Input: part model. Units: mm. Frame: model coordinates. Coordinates: 2 decimals unless noted, no trailing zeros. Loops run counter-clockwise (first coordinate to the right, second up) from the corner with the lowest first, then second, coordinate; pieces in that order, holes last.
```python
from build123d import *

# Parameters (mm, degrees)
SKETCH093_W      = 26
SKETCH093_H      = 70
EXTRUDE081_DEPTH = 1
SKETCH_W         = 45
SKETCH_H         = 66
EXTRUDE_DEPTH    = 2


with BuildPart() as extrude081:
    # Sketch093 → Extrude081 (new body, symmetric)
    with BuildSketch(Plane.XY.offset(-22)):
        with Locations((62, 50)):
            Rectangle(SKETCH093_W, SKETCH093_H)
    extrude(amount=EXTRUDE081_DEPTH, both=True)


with BuildPart() as cut012:
    # Sketch → Extrude (new body)
    with BuildSketch(Plane(origin=(0, 0, -22), x_dir=(1, 0, 0), z_dir=(0, 0, -1))):
        Polygon((-7, 2), (81, 2), (81, -102), (-7, -102), (-7, -100), (-2, -100), (-2, -93.5), (-3, -93.5), (-3, -9), (-2, -9), (-2, 0), (-7, 0), align=None)
        with Locations((20.5, -52)):
            Rectangle(SKETCH_W, SKETCH_H, mode=Mode.SUBTRACT)
    extrude(amount=EXTRUDE_DEPTH)

    # Cut012: cut Extrude081
    add(extrude081.part, mode=Mode.SUBTRACT)


solid = cut012.part
```
Item 1: Line query: L1, parallel to X at y = 20.5, z = -22.05; L2, parallel to Y at x = 6, z = -23.2; L3, parallel to X at y = 26, z = -23.85. Output: solid intervals per line, ascending.
Result:
L1: x = -3 to -2, 43 to 49, 75 to 81
L2: y = -2 to 19, 85 to 102
L3: x = -3 to -2, 43 to 81
Item 2: Section query B-B (z = -23.55). Output: boundary loops of the cut face in (x, y).
Result:
outline: (-7, -2) - (81, -2) - (81, 102) - (-7, 102) - (-7, 100) - (-2, 100) - (-2, 93.5) - (-3, 93.5) - (-3, 9) - (-2, 9) - (-2, 0) - (-7, 0) - close; hole (-2, 19) - (43, 19) - (43, 85) - (-2, 85) - close
Item 3: Mould query, pull axis Y, two halves, no side actions, for faces 1 (the face through (62, 50, -23)), 2 (the face through (47, 38, -22)). Classes: +Y half, -Y half, draft (parallel to the pull), parting line (faces both ways), or undercut.
Result:
face 1: undercut
face 2: draft
Item 4: Contact query for flat-ended pins moving along their axis: P1, Ø6, axis at x = 64, y = 44.5, coming from the +Z side; P2, Ø0.5, axis at y = 66.5, z = -22.5, coming from the -X side; P3, Ø0.6, axis at y = 95.5, z = -22.5, coming from the -X side. Output: stop coordinate, or through.
Result:
P1: stops at z = -23
P2: stops at x = -3
P3: stops at x = -2
Item 5: Section query A-A (y = 60.5). Output: boundary loops of the cut face in (x, z), then the cut area to 3 significant figures.
Result:
outline: (-3, -24) - (-2, -24) - (-2, -22) - (-3, -22) - close; (43, -24) - (81, -24) - (81, -22) - (75, -22) - (75, -23) - (49, -23) - (49, -22) - (43, -22) - close
area: 52.0 mm2
Item 6: Section query D-D (x = 55). Output: boundary loops of the cut face in (y, z), then the cut area to 3 significant figures.
Result:
outline: (-2, -24) - (102, -24) - (102, -22) - (85, -22) - (85, -23) - (15, -23) - (15, -22) - (-2, -22) - close
area: 138 mm2
Item 7: Section query C-C (x = 16). Output: boundary loops of the cut face in (y, z).
Result:
outline: (-2, -24) - (19, -24) - (19, -22) - (-2, -22) - close; (85, -24) - (102, -24) - (102, -22) - (85, -22) - close
